Can you work these out from the model? Positions are in its coordinate system, mm. A direction names the side the tool comes from. Coordinates: 2 decimals unless noted, no trailing zeros. Write each loop counter-clockwise with the first axis right and the second up, starting at its lowest first coordinate (ties: lowest second). Pieces come first, ordered by that corner, then holes. Notation, with made-up numbers: (86, 25.5) -> (103, 25.5) arc R23 cw to (103, 44.5) -> close; hole circle Ø3 at (-35, 1). An arc over 180 degrees is marked (long way). Use one line per item in the form item = value.
```python
from build123d import *

# Parameters (mm, degrees)
CROQUIS1_W              = 569.383333334
CROQUIS1_H              = 369.485333334
SALIENTE_EXTRUIR1_DEPTH = 25.4
VACIADO1_T              = -3.175
CROQUIS2_R              = 3.96875
SALIENTE_EXTRUIR2_DEPTH = 4.7625


with BuildPart() as part:
    # Croquis1 → Saliente-Extruir1 (new body)
    with BuildSketch(Plane(origin=(0, 0, 0), x_dir=(1, 0, 0), z_dir=(0, 1, 0))):
        with Locations((327.025, 227.076)):
            Rectangle(CROQUIS1_W, CROQUIS1_H)
    extrude(amount=SALIENTE_EXTRUIR1_DEPTH)

    # Vaciado1
    vaciado1_openings = [part.faces().sort_by_distance(p)[0] for p in [
        (327.025, 0, -227.076),
    ]]
    offset(amount=VACIADO1_T, openings=vaciado1_openings, kind=Kind.INTERSECTION)

    # Croquis2 → Saliente-Extruir2 (add)
    with BuildSketch(Plane(origin=(611.716666667, 0, 0), x_dir=(0, 0, -1), z_dir=(1, 0, 0))):
        with BuildLine():
            Line((411.818666667, 0), (411.818666667, 25.4))
            Line((411.818666667, 25.4), (432.983666667, 25.4))
            ThreePointArc((432.983666667, 25.4), (439.333666667, 19.05), (432.983666667, 12.7))
            ThreePointArc((432.983666667, 12.7), (421.536041367, 9.233937949), (413.933666667, 0))
            Line((413.933666667, 0), (411.818666667, 0))
        make_face()
        with Locations((432.983666667, 19.05)):
            Circle(CROQUIS2_R, mode=Mode.SUBTRACT)
    saliente_extruir2 = extrude(amount=-SALIENTE_EXTRUIR2_DEPTH)

    # Simetría1: Saliente-Extruir2 across plane
    add(saliente_extruir2.mirror(Plane(origin=(327.025, 0, 0), x_dir=(0, 0, 1), z_dir=(1, 0, 0))))


solid = part.part
```
Q1. For faces 1 (the flat face through (606.954, 16, -423)), 2 (the cylindrical face through (44.68, 9.33, -421.68)), 3 (the flat face through (323, 22.225, -230)), which set-ups out of +Z, -Z, +X, -X, +Y, -Y let a thin tool reach every point of the face, with its end or its side?
Return value:
face_1 = -Z, +Y, -Y
face_2 = -Z, +X, -X, -Y
face_3 = -Y
Q2. Suppose I cut it at C-C (x = 269). Write out the boundary of the cut face in (y, z) (3 decimals), then the cut area to 3 significant figures.
Return value:
outline = (0, -411.819) -> (25.4, -411.819) -> (25.4, -42.333) -> (0, -42.333) -> (0, -45.508) -> (22.225, -45.508) -> (22.225, -408.644) -> (0, -408.644) -> close
area = 1,310 mm2
Q3. Will these pins go through, and if not, where does the flat tip stop? pin 1 (1.5 mm diameter, centred on x = 537, z = -255.5, fed in from -Y) (3 decimals); pin 2 (12.5 mm diameter, centred on x = 414, y = 11, fed in from -Z).
Return value:
pin_1 = 22.225
pin_2 = -411.82
Q4. Suppose I cut it at B-B (y = 6.5). Write out the boundary of the cut face in (x, z).
Return value:
outline = (42.33, -418.24) -> (47.1, -418.24) -> (47.1, -411.82) -> (606.95, -411.82) -> (606.95, -418.24) -> (611.72, -418.24) -> (611.72, -42.33) -> (42.33, -42.33) -> close; hole (45.51, -408.64) -> (608.54, -408.64) -> (608.54, -45.51) -> (45.51, -45.51) -> close
Q5. If I drill on line 1 (Z direction, x = 414.5, y = 8.5); line 2 (X direction, y = 21.5, z = -284); line 3 (Y direction, x = 487, z = -106.5) (3 decimals), over which ranges is the centre line in solid material (lowest first)? Write a range as from..to.
Return value:
line_1 = -411.82..-408.64, -45.51..-42.33
line_2 = 42.33..45.51, 608.54..611.72
line_3 = 22.225..25.4
Q6. Suppose I cut it at A-A (z = -234.5). Write out the boundary of the cut face in (x, y) (3 decimals), then the cut area to 3 significant figures.
Return value:
outline = (42.333, 0) -> (45.508, 0) -> (45.508, 22.225) -> (608.542, 22.225) -> (608.542, 0) -> (611.717, 0) -> (611.717, 25.4) -> (42.333, 25.4) -> close
area = 1,950 mm2
Q7. Thinking about a two-plate mould opening in Z: for faces 4 (the flat face through (323, 11, -408.644)), 5 (the flat face through (45.508, 11, -225)), 6 (the flat face through (47.096, 16, -423)), 7 (the flat face through (323, 13, -411.819)), which applies, released by +Z, released by -Z, zero draft, split by the parting line, or undercut?
Return value:
face_4 = undercut
face_5 = undercut
face_6 = zero draft
face_7 = released by -Z
